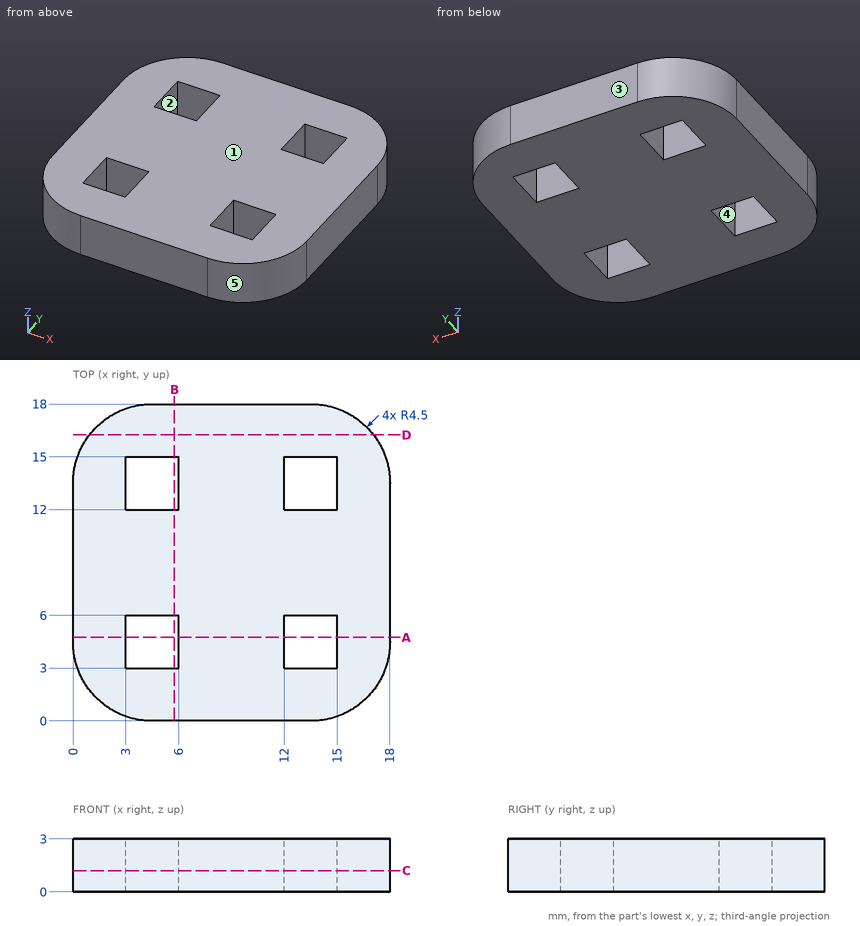
Job drawing, mm, ordinate dimensions from the low corner. One solid piece. A direction names the side the tool comes from. Give positions to 0.01 mm unless a question says otherwise; leave off trailing zeros. Loops run counter-clockwise (first coordinate to the right, second up) from the corner with the lowest first, then second, coordinate; pieces in that order, holes last. Notation, with made-up numbers: (75, 7) -> (102, 7) arc R28 ccw to (102, 33) -> close; hole circle Ø9 at (-8.5, -39.5). An arc over 180 degrees is marked (long way). Write each question's results on one line, items separated by ' | '. Start each with the question number.
Q1. Band-saw the part on D-D on y = 16.25. List the corners of the cut face in (x, z), plus the area to 3 significant figures.
Q2. Band-saw the part on A-A on y = 4.75. List the corners of the cut face in (x, z), plus the area to 3 significant figures.
Q3. Which spindle directions (+Z, -Z, +X, -X, +Y, -Y) get a long thin tool onto all of the face, cutting with end or side? Do the marked faces 1 and 2. Say none if no direction does.
Q4. Pull direction Y, two halves, no side cores. Call the marked faces 3, 4 and 5: +Y half, -Y half, draft (parallel to the pull), parting line (faces both ways), or undercut.
Q5. Wall check: L1, parallel to Y at x = 5.75, z = 1.85; L2, parallel to Y at x = 3.25, z = 1.9. Give the ranges that are in metal, low to high.
Q6. Band-saw the part on C-C on z = 1.2. List the corners of the cut face in (x, y), plus the area to 3 significant figures.
Results are:
1) outline: (0.94, 0) -> (17.06, 0) -> (17.06, 3) -> (0.94, 3) -> close | area: 48.4 mm²
2) outline: (0, 0) -> (3, 0) -> (3, 3) -> (0, 3) -> close; (6, 0) -> (12, 0) -> (12, 3) -> (6, 3) -> close; (15, 0) -> (18, 0) -> (18, 3) -> (15, 3) -> close | area: 36.0 mm²
3) face 1: +Z, +X, -X, +Y, -Y | face 2: +Z, -Z
4) face 3: +Y half | face 4: undercut | face 5: -Y half
5) L1: y = 0 to 3, 6 to 12, 15 to 18 | L2: y = 0.18 to 3, 6 to 12, 15 to 17.82
6) outline: (0, 4.5) arc R4.5 ccw to (4.5, 0) -> (13.5, 0) arc R4.5 ccw to (18, 4.5) -> (18, 13.5) arc R4.5 ccw to (13.5, 18) -> (4.5, 18) arc R4.5 ccw to (0, 13.5) -> close; hole (3, 3) -> (6, 3) -> (6, 6) -> (3, 6) -> close; hole (3, 12) -> (6, 12) -> (6, 15) -> (3, 15) -> close; hole (12, 3) -> (15, 3) -> (15, 6) -> (12, 6) -> close; hole (12, 12) -> (15, 12) -> (15, 15) -> (12, 15) -> close | area: 271 mm²
